```python
from build123d import *

# Parameters (mm, degrees)
ESBO_O1_R                = 3.5
ESBO_O1_R_2              = 1.5
RESSALTO_EXTRUS_O1_DEPTH = 3


with BuildPart() as part:
    # Esboço1 → Ressalto-extrusão1 (new body)
    with BuildSketch(Plane(origin=(0, 0, 0), x_dir=(1, 0, 0), z_dir=(0, 1, 0))):
        with BuildLine():
            Line((-1.543118166, -51.877133975), (-2.882093194, -43.377133975))
            ThreePointArc((-2.882093194, -43.377133975), (-5.555698335, -21.698089912), (-6.543118166, 0.122866025))
            ThreePointArc((-6.543118166, 0.122866025), (-5.322348439, 9.715942783), (-0.543118166, 18.122866025))
            ThreePointArc((-0.543118166, 18.122866025), (-0.043118166, 18.346048676), (0.456881834, 18.122866025))
            ThreePointArc((0.456881834, 18.122866025), (5.236112108, 9.715942783), (6.456881834, 0.122866025))
            ThreePointArc((6.456881834, 0.122866025), (5.469462003, -21.698089912), (2.795856862, -43.377133975))
            Line((2.795856862, -43.377133975), (1.456881834, -51.877133975))
            ThreePointArc((1.456881834, -51.877133975), (-0.043118166, -53.479108362), (-1.543118166, -51.877133975))
        make_face()
        with Locations(Location((-0.043118166, 0.122866025, 0), (0, 0, 270))):
            Circle(ESBO_O1_R, mode=Mode.SUBTRACT)
        with Locations(Location((-0.043118166, -24.377133975, 0), (0, 0, 270))):
            Circle(ESBO_O1_R_2, mode=Mode.SUBTRACT)
        with Locations(Location((-0.043118166, -43.377133975, 0), (0, 0, 270))):
            Circle(ESBO_O1_R_2, mode=Mode.SUBTRACT)
        Polygon((-0.043118166, -14.877133975), (-0.543118166, -14.877133975), (-0.543118166, -8.877133975), (0.456881834, -8.877133975), (0.456881834, -14.877133975), align=None, mode=Mode.SUBTRACT)
        Polygon((0.456881834, 15.122866025), (-0.043118166, 15.122866025), (-0.543118166, 15.122866025), (-0.543118166, 9.122866025), (0.456881834, 9.122866025), align=None, mode=Mode.SUBTRACT)
        Polygon((-0.043118166, -28.877133975), (1.456881834, -28.877133975), (1.456881834, -38.877133975), (-0.043118166, -38.877133975), (-1.543118166, -38.877133975), (-1.543118166, -28.877133975), align=None, mode=Mode.SUBTRACT)
    extrude(amount=RESSALTO_EXTRUS_O1_DEPTH)


solid = part.part
```
Model file for the job. Use its own axes, mm. A direction names the side the tool comes from. Coordinates: 2 decimals unless noted, no trailing zeros. Write each loop counter-clockwise with the first axis right and the second up, starting at its lowest first coordinate (ties: lowest second). Pieces come first, ordered by that corner, then holes. Notation, with made-up numbers: (-34, 11) - (-17, 11) arc R27 ccw to (-17, 47) - close; hole circle Ø3 at (66.25, -36.5). An arc over 180 degrees is marked (long way). Use a Markdown table: item, result. Add a question column.
Item 1: Two-plate mould, pull along X, no slides. Class faces 3 (the face through (0, 0, 17)), 4 (the face through (5.495, 1.479, 21.393)), 5 (the face through (-5.53, 1.48, 22)), 6 (the face through (0, 1, 38.877)): pulls with the +X half, pulls with the -X half, needs draft (parallel to the pull), parting line crosses it, or undercut.
Item 2: Drill centre lines: line 1 along X through (y, z) = (0.1, 44.5); line 2 along X through (y, z) = (2.8, 11); line 3 along X through (y, z) = (0.1, 5.5). Where is each one in solid material? Low to high.
Item 3: Band-saw the part on B-B, the plane y = 0.6. Write the cut outline in (x, z).
Item 4: Band-saw the part on A-A, the plane z = 32. Write the cut outline in (x, y), and give its area (3 significant figures).
Item 5: 3-axis set-ups, long thin cutter, end or side, ignore diameter. For faces 1 (the face through (0.457, 1, 12)), 2 (the face through (0, 3, 17)): which of +Z, -Z, +X, -X, +Y, -Y reach the whole face in a straight line?
Item 6: Drop flat-ended pins along their axis: pin 1 (0.9 mm diameter, centred on y = 1.5, z = -13, fed in from -X); pin 2 (2.5 mm diameter, centred on x = -0.04, z = 24.38, fed in from +Y). Give the stop position or say it passes through.
Item 7: Band-saw the part on D-D, the plane z = -7. Write the cut outline in (x, y).
A:
| question | item | result |
|---|---|---|
| 1 | face 3 | needs draft |
| 1 | face 4 | pulls with the +X half |
| 1 | face 5 | pulls with the -X half |
| 1 | face 6 | undercut |
| 2 | line 1 | x = -2.71 to -1.04, 0.95 to 2.62 |
| 2 | line 2 | x = -6.25 to -0.54, 0.46 to 6.17 |
| 2 | line 3 | x = -6.45 to 6.36 |
| 3 | outline | (-6.54, -0.12) arc R24.93 ccw to (-0.54, -18.12) arc R0.67 ccw to (0.46, -18.12) arc R24.93 ccw to (6.46, -0.12) arc R281.97 ccw to (2.8, 43.38) - (1.46, 51.88) arc R1.5 ccw (long way) to (-1.54, 51.88) - (-2.88, 43.38) arc R281.97 ccw to start; hole circle Ø7 at (-0.04, -0.12); hole circle Ø3 at (-0.04, 24.38); hole (-1.54, 28.88) - (1.46, 28.88) - (1.46, 38.88) - (-1.54, 38.88) - close; hole circle Ø3 at (-0.04, 43.38); hole (-0.54, -15.12) - (0.46, -15.12) - (0.46, -9.12) - (-0.54, -9.12) - close; hole (-0.54, 8.88) - (0.46, 8.88) - (0.46, 14.88) - (-0.54, 14.88) - close |
| 4 | outline | (-4.5, 0) - (-1.54, 0) - (-1.54, 3) - (-4.5, 3) - close; (1.46, 0) - (4.41, 0) - (4.41, 3) - (1.46, 3) - close |
| 4 | area | 17.7 mm² |
| 5 | face 1 | +Y, -Y |
| 5 | face 2 | +Z, -Z, +X, -X, +Y |
| 6 | pin 1 | stops at x = -4.18 |
| 6 | pin 2 | passes through |
| 7 | outline | (-6.06, 0) - (5.97, 0) - (5.97, 3) - (-6.06, 3) - close |
